```python
from build123d import *

# Parameters (mm, degrees)
SKETCH_1_R      = 1.25
EXTRUDE_1_DEPTH = 16
CHAMFER_1_SIZE  = 0.3
SKETCH_2_R      = 1.55
EXTRUDE_2_DEPTH = 2
EXTRUDE_START   = 3
SKETCH_3_R      = 1.25
EXTRUDE_3_DEPTH = 3


with BuildPart() as part:
    # 草图1 → 凸台-拉伸1 (new body)
    with BuildSketch(Plane.YZ):
        Polygon((2.655811238, 0), (1.327905619, 2.3), (-1.327905619, 2.3), (-2.655811238, 0), (-1.327905619, -2.3), (1.327905619, -2.3), align=None)
        with Locations(Location((0, 0, 0), (0, 0, 270))):
            Circle(SKETCH_1_R, mode=Mode.SUBTRACT)
    extrude(amount=EXTRUDE_1_DEPTH)

    # 倒角1
    chamfer_1_edges = [part.edges().sort_by_distance(p)[0] for p in [
        (16, 0, 2.3),
        (16, -1.991858429, 1.15),
        (0, 0, 1.25),
        (16, 0, 1.25),
        (16, -1.991858429, -1.15),
        (16, 0, -2.3),
        (16, 1.991858429, -1.15),
        (0, 0, -2.3),
        (0, -1.991858429, -1.15),
        (0, -1.991858429, 1.15),
        (0, 0, 2.3),
        (0, 1.991858429, 1.15),
        (0, 1.991858429, -1.15),
        (16, 1.991858429, 1.15),
    ]]
    chamfer(chamfer_1_edges, length=CHAMFER_1_SIZE)

    # 草图2 → 凸台-拉伸2 (add)
    with BuildSketch(Plane.ZY):
        Circle(SKETCH_2_R)
    extrude(amount=-EXTRUDE_2_DEPTH)

    # 草图3 → 凸台-拉伸3 (add)
    with BuildSketch(Plane.ZY.offset(EXTRUDE_START)):
        Circle(SKETCH_3_R)
    extrude(amount=-EXTRUDE_3_DEPTH)


solid = part.part
```
CAD build for the part. Positions are in the model's coordinates, mm. A direction names the side the tool comes from. Give positions to 0.01 mm unless a question says otherwise; leave off trailing zeros. Loops run counter-clockwise (first coordinate to the right, second up) from the corner with the lowest first, then second, coordinate; pieces in that order, holes last. Notation, with made-up numbers: (50, 48) -> (70, 48) arc R19 ccw to (70, 80) -> close; hole circle Ø2 at (-4.5, 63). An arc over 180 degrees is marked (long way). Use a Markdown table: item, result.
1. Slice it at B-B (y = 0). List the corners of the cut face in (x, z).
Check result:
| item | result |
|---|---|
| outline | (-3, -1.25) -> (0, -1.25) -> (0, -2) -> (0.3, -2.3) -> (15.7, -2.3) -> (16, -2) -> (16, -1.55) -> (15.7, -1.25) -> (2, -1.25) -> (2, 1.25) -> (15.7, 1.25) -> (16, 1.55) -> (16, 2) -> (15.7, 2.3) -> (0.3, 2.3) -> (0, 2) -> (0, 1.25) -> (-3, 1.25) -> close |
2. Wall check: L1, parallel to Z at x = 9.25, y = 0; L2, parallel to X at y = -0.15, z = 1.2; L3, parallel to X at y = 1.75, z = 0.85. Give the ranges that are in metal, low to high. Write a range as [from, to].
Check result:
| item | result |
|---|---|
| L1 | z = [-2.3, -1.25], [1.25, 2.3] |
| L2 | x = [-3, 2] |
| L3 | x = [0, 16] |
3. Mould opens along Z. For faces 3 (the flat face through (-3, 0, 0)), 4 (the flat face through (7.892, 2.001, 1.134)), 5 (the flat face through (2, 0, 0)) say: pulls with the +Z half, pulls with the -Z half, needs draft (parallel to the pull), parting line crosses it, or undercut.
Check result:
| item | result |
|---|---|
| face 3 | needs draft |
| face 4 | pulls with the +Z half |
| face 5 | undercut |
4. Slice it at A-A (x = 4.5). List the corners of the cut face in (y, z).
Check result:
| item | result |
|---|---|
| outline | (-2.66, 0) -> (-1.33, -2.3) -> (1.33, -2.3) -> (2.66, 0) -> (1.33, 2.3) -> (-1.33, 2.3) -> close; hole circle Ø2.5 at (0, 0) |
5. Which spindle directions (+Z, -Z, +X, -X, +Y, -Y) get a long thin tool onto all of the face, cutting with end or side? Do faces 1 (the cylindrical face through (-1.52, -1.22, -0.27)), 2 (the flat face through (15.852, 1.851, -1.09)). Say none if no direction does.
Check result:
| item | result |
|---|---|
| face 1 | -X |
| face 2 | -Z, +X, +Y |
6. Slice it at C-C (z = -1.75). List the corners of the cut face in (x, y), plus the area to 3 significant figures.
Check result:
| item | result |
|---|---|
| outline | (0, -1.3) -> (0.3, -1.65) -> (15.7, -1.65) -> (16, -1.3) -> (16, 1.3) -> (15.7, 1.65) -> (0.3, 1.65) -> (0, 1.3) -> close |
| area | 52.4 mm^2 |
7. Slice it at D-D (x = -1). List the corners of the cut face in (y, z), plus the area to 3 significant figures.
Check result:
| item | result |
|---|---|
| outline | circle Ø2.5 at (0, 0) |
| area | 4.91 mm^2 |
8. Flat gauge pins, fed straight in: pin 1 (1 mm diameter, centred on x = 11.5, z = -1, fed in from -Y); pin 2 (1.5 mm diameter, centred on y = 0, z = 0, fed in from +X); pin 3 (1.2 mm diameter, centred on y = 0.5, z = 0.5, fed in from +X). Where does each tip first touch, or does it go through?
Check result:
| item | result |
|---|---|
| pin 1 | stops at y = -2.37 |
| pin 2 | stops at x = 2 |
| pin 3 | stops at x = 15.76 |
